```python
from build123d import *

# Parameters (mm, degrees)
F1_DEPTH = 100
F2_R     = 25
F3_DEPTH = 30
F4_R     = 25
F5_DEPTH = 25
F7_DEPTH = 30


with BuildPart() as f1:
    # F0 (on Front) → F1 (new body)
    with BuildSketch(Plane.XZ):
        Polygon((125, 50), (-125, 50), (-150, 50), (-125, -50), (125, -50), (150, 50), align=None)
    extrude(amount=-F1_DEPTH)

    # F2 (on face) → F3 (join)
    with BuildSketch(Plane.XZ):
        Polygon((125, -50), (150, 50), (-150, 50), (-125, -50), align=None)
        with Locations((-50, 0)):
            Circle(F2_R, mode=Mode.SUBTRACT)
        with BuildLine():
            ThreePointArc((25, 0), (50, 25), (75, 0))
            ThreePointArc((75, 0), (50, -25), (25, 0))
        make_face(mode=Mode.SUBTRACT)
    extrude(amount=F3_DEPTH)

    # F4 (on face) → F5 (cut)
    with BuildSketch(Plane.XY.offset(50)):
        with Locations((0, 50.720426)):
            Circle(F4_R)
    extrude(amount=-F5_DEPTH, mode=Mode.SUBTRACT)

    # F6 (on face) → F7 (cut)
    with BuildSketch(Plane(origin=(0, 100, 0), x_dir=(-1, 0, 0), z_dir=(0, 1, 0))):
        with BuildLine():
            Line((-25, -50), (0, -50))
            Line((0, -50), (25, -50))
            Line((25, -50), (25, -25))
            ThreePointArc((25, -25), (23.535534, -21.464466), (20, -20))
            Line((20, -20), (-20, -20))
            ThreePointArc((-20, -20), (-23.535534, -21.464466), (-25, -25))
            Line((-25, -25), (-25, -50))
        make_face()
    extrude(amount=-F7_DEPTH, mode=Mode.SUBTRACT)


solid = f1.part
```
Design review of the part built by this model. Coordinates are the model's own, in mm. A direction names the side the tool comes from. Round coordinates to 2 decimals unless told otherwise and drop trailing zeros. Order: outer loops, then holes, each group sorted by start corner. A loop starts at its lowest first (then second) coordinate and runs counter-clockwise, first axis right, second up. Notation, with made-up numbers: (66, 64.25) - (92, 64.25) arc R18 cw to (92, 70.25) - close; hole circle Ø5 at (56, -8). An arc over 180 degrees is marked (long way). Return JSON: item names as keys, results as strings.
Q1. The part is to be moulded in two halves that separate along X. For faces 4 (the flat face through (137.325, 35.91, -0.7)), 5 (the flat face through (2, 21, 50)), 6 (the cylindrical face through (-5.42, 26.315, 37.675)), 7 (the cylindrical face through (30, -15, 15)), say which applies: pulls with the +X half, pulls with the -X half, needs draft (parallel to the pull), parting line crosses it, or undercut.
Computed values:
{"face 4": "pulls with the +X half", "face 5": "needs draft", "face 6": "undercut", "face 7": "undercut"}
Q2. For pin 1 Ø2 at (y, z) = (23, -25.5) entering from -X (3 decimals); pin 2 Ø8 at (x, z) = (-5.5, -24.5) entering from +Y; pin 3 Ø12 at (y, z) = (40.5, 2) entering from +X, all flat-tipped, find the tip position at first contact; note any pin that passes through.
Computed values:
{"pin 1": "stops at x = -131.375", "pin 2": "stops at y = 70", "pin 3": "stops at x = 139.5"}
Q3. Consider section A-A on z = -15. Write out the cut boundary in (x, y).
Computed values:
{"outline": "(-133.75, -30) - (-70, -30) - (-70, 0) - (-30, 0) - (-30, -30) - (30, -30) - (30, 0) - (70, 0) - (70, -30) - (133.75, -30) - (133.75, 100) - (-133.75, 100) - close"}
Q4. Machinability: for faces 1 (the flat face through (-25, 85, -38)), 2 (the flat face through (50, 0, 0)), 3 (the flat face through (0, 51, 25)), which of the approach directions +Z, -Z, +X, -X, +Y, -Y give a long, thin tool a straight path to every point of the face, cutting with its end or side? Answer none if there is none.
Computed values:
{"face 1": "-Z, +Y", "face 2": "-Y", "face 3": "+Z"}
Q5. Consider section B-B on x = 0. Write out the cut boundary in (y, z).
Computed values:
{"outline": "(-30, -50) - (70, -50) - (70, -20) - (100, -20) - (100, 50) - (75.72, 50) - (75.72, 25) - (25.72, 25) - (25.72, 50) - (-30, 50) - close"}
Q6. Wall thickness on L1, parallel to Y at x = 0, z = 39; L2, parallel to X at y = -2, z = -11; L3, parallel to Y at x = 45.5, z = 6: over which ranges is each line inside the solid? List them lowest first. Write a range as [from, to].
Computed values:
{"L1": "y = [-30, 25.72], [75.72, 100]", "L2": "x = [-134.75, -72.45], [-27.55, 27.55], [72.45, 134.75]", "L3": "y = [0, 100]"}
Q7. Consider section D-D on x = 50. Write out the cut boundary in (y, z).
Computed values:
{"outline": "(-30, -50) - (100, -50) - (100, 50) - (-30, 50) - (-30, 25) - (0, 25) - (0, -25) - (-30, -25) - close"}
Q8. Consider section C-C on y = -12. Write out the cut boundary in (x, z).
Computed values:
{"outline": "(-150, 50) - (-125, -50) - (125, -50) - (150, 50) - close; hole circle Ø50 at (-50, 0); hole circle Ø50 at (50, 0)"}
